Model file for the job. Use its own axes, mm. Round coordinates to 2 decimals unless told otherwise and drop trailing zeros. Order: outer loops, then holes, each group sorted by start corner. A loop starts at its lowest first (then second) coordinate and runs counter-clockwise, first axis right, second up. Notation, with made-up numbers: (38, 25) - (58, 25) arc R14 ccw to (58, 35) - close; hole circle Ø11 at (18.5, 66). An arc over 180 degrees is marked (long way). Answer as CSV lines item,"result". Start each with the question number.
1. Band-saw the part on A-A on x = 16. List the corners of the cut face in (y, z), then the cut area to 3 significant figures.
2. Pin check, flat tips, straight feed: pin 1 Ø1 at (y, z) = (0.5, 1) entering from +X; pin 2 Ø0.6 at (y, z) = (0.5, 9.5) entering from -X; pin 3 Ø2 at (x, z) = (8, 0) entering from -Y; pin 4 Ø0.6 at (y, z) = (1, 14.5) entering from +X. Stop position of each tip, or through.
3. Band-saw the part on B-B on z = -2.25. List the corners of the cut face in (x, y).
4. Wall check: line 1 along X through (y, z) = (1.1, 0); line 2 along X through (y, z) = (0.3, -0.25); line 3 along Z through (x, y) = (15, 1.45). Give the ranges that are in metal, low to high. Write a range as [from, to].
5. Band-saw the part on C-C on x = 4. List the corners of the cut face in (y, z), then the cut area to 3 significant figures.
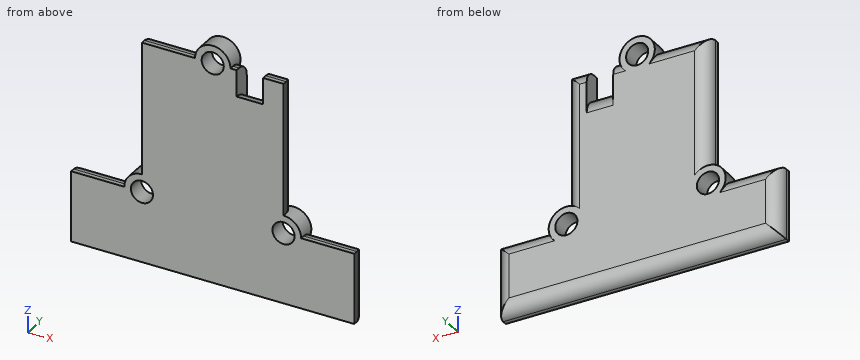
```python
from build123d import *

# Parameters (mm, degrees)
ESQUISSE1_W             = 32
ESQUISSE1_H             = 8
BOSS_EXTRU_1_DEPTH      = 2
BOSS_EXTRU_2_DEPTH      = 2
ESQUISSE3_R             = 1.9999999999999996
ESQUISSE3_R_2           = 2.000000000000003
ESQUISSE3_R_3           = 1.9999999999999991
BOSS_EXTRU_3_DEPTH      = 2
ESQUISSE4_R             = 1.2499999999999991
ESQUISSE4_R_2           = 1.250000000000001
ESQUISSE4_R_3           = 1.2500000000000013
ENL_V_MAT_EXTRU_1_DEPTH = 2
CONG_1_R                = 1.5
ENL_V_MAT_EXTRU_2_DEPTH = 38.26929044937668
CONG_2_R                = 2


with BuildPart() as part:
    # Esquisse1 → Boss.-Extru.1 (new body)
    with BuildSketch(Plane(origin=(0, 0, 0), x_dir=(1, 0, 0), z_dir=(0, 1, 0))):
        with Locations((16, 4)):
            Rectangle(ESQUISSE1_W, ESQUISSE1_H)
    extrude(amount=BOSS_EXTRU_1_DEPTH)

    # Esquisse2 → Boss.-Extru.2 (add)
    with BuildSketch(Plane(origin=(0, 2, 0), x_dir=(1, 0, 0), z_dir=(0, 1, 0))):
        Polygon((8.000000000000002, 4.5e-16), (24, 2.41e-15), (24.000000000000004, -17), (8.000000000000004, -17), align=None)
    extrude(amount=-BOSS_EXTRU_2_DEPTH)

    # Esquisse3 → Boss.-Extru.3 (add)
    with BuildSketch(Plane(origin=(0, 2, 0), x_dir=(1, 0, 0), z_dir=(0, 1, 0))):
        with Locations((8.000000000000002, 0)):
            Circle(ESQUISSE3_R)
        with Locations((24, 2.41e-15)):
            Circle(ESQUISSE3_R_2)
        with Locations((16.000000000000004, -17)):
            Circle(ESQUISSE3_R_3)
    extrude(amount=-BOSS_EXTRU_3_DEPTH)

    # Esquisse4 → Enlèv. mat.-Extru.1 (cut)
    with BuildSketch(Plane(origin=(0, 2, 0), x_dir=(1, 0, 0), z_dir=(0, 1, 0))):
        with Locations(Location((8.000000000000002, 0, 0), (0, 0, 270))):
            Circle(ESQUISSE4_R)
        with Locations(Location((24, 2.41e-15, 0), (0, 0, 270))):
            Circle(ESQUISSE4_R_2)
        with Locations(Location((16.000000000000004, -17, 0), (0, 0, 270))):
            Circle(ESQUISSE4_R_3)
    extrude(amount=-ENL_V_MAT_EXTRU_1_DEPTH, mode=Mode.SUBTRACT)

    # Congé1
    cong_1_edges = [part.edges().sort_by_distance(p)[0] for p in [
        (32, 2, -4),
        (16, 2, -8),
        (11.000000000000004, 2, 17),
        (24.000000000000004, 2, 9.500000000000002),
        (8.000000000000004, 2, 9.5),
        (29, 2, 0),
        (0, 2, -4),
        (21.000000000000004, 2, 17),
        (3.000000000000001, 2, 0),
    ]]
    fillet(cong_1_edges, radius=CONG_1_R)

    # Esquisse5 → Enlèv. mat.-Extru.2 (cut, through all)
    with BuildSketch(Plane.XZ):
        Polygon((21.700000000000003, 17), (18.700000000000003, 17), (18.70000000000001, 14.000000000000002), (21.700000000000006, 14.000000000000002), align=None)
    extrude(amount=-ENL_V_MAT_EXTRU_2_DEPTH, mode=Mode.SUBTRACT)

    # Congé2
    cong_2_edges = [part.edges().sort_by_distance(p)[0] for p in [
        (20.20000000000001, 2, 14),
    ]]
    fillet(cong_2_edges, radius=CONG_2_R - 0.0001)  # a hair under: the kernel refuses the full size


solid = part.part
```
Reply:
1,outline,"(0, -8) - (0.5, -8) arc R1.5 ccw to (2, -6.5) - (2, 15.75) - (0, 15.75) - close; (0, 18.25) - (2, 18.25) - (2, 19) - (0, 19) - close"
1,area,"48.5 mm2"
2,pin 1,"stops at x = 25.94"
2,pin 2,"stops at x = 8"
2,pin 3,"passes through"
2,pin 4,"stops at x = 23.99"
3,outline,"(0, 0) - (32, 0) - (32, 0.5) arc R1.5 ccw to (30.5, 2) - (1.5, 2) arc R1.5 ccw to (0, 0.5) - close"
4,line 1,"x = [6, 6.75], [9.25, 22.75], [25.25, 26]"
4,line 2,"x = [0, 6.78], [9.22, 22.78], [25.22, 32]"
4,line 3,"z = [-7.66, 16.25], [17.75, 18.73]"
5,outline,"(0, -8) - (0.5, -8) arc R1.5 ccw to (2, -6.5) - (2, -1.5) arc R1.5 ccw to (0.5, 0) - (0, 0) - close"
5,area,"15.0 mm2"
